Check sheet for the drawn part. Datum: minimum x, y, z corner. Units: mm. A direction names the side the tool comes from. Round coordinates to 2 decimals unless told otherwise and drop trailing zeros. Order: outer loops, then holes, each group sorted by start corner. A loop starts at its lowest first (then second) coordinate and runs counter-clockwise, first axis right, second up. Notation, with made-up numbers: (20, 30) -> (66, 30) arc R25 cw to (66, 60) -> close; hole circle Ø6 at (52, 80). An arc over 180 degrees is marked (long way). Answer as CSV lines item,"result". Start each with the question number.
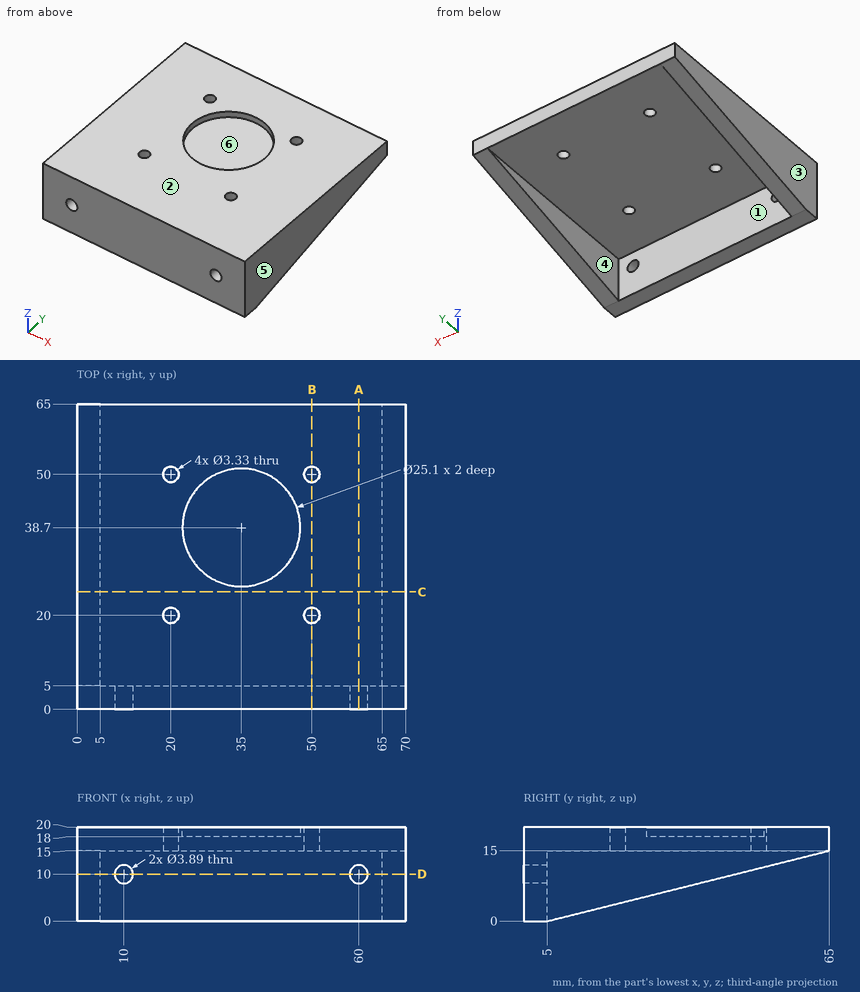
1) Section check B-B on x = 50. Record the cut outline in (y, z) (3 decimals), then the cut area to 3 significant figures.
2) Mould release check, pull along X, two halves, no side actions. Record for the marked faces 1, 2 and 3: released by +X, released by -X, zero draft, split by the parting line, or undercut.
3) Material ranges on line 1 along X through (y, z) = (20, 18.1) (3 decimals); line 2 along Y through (x, z) = (50, 18.9) (3 decimals); line 3 along Z through (x, y) = (60, 3.45) (3 decimals), recorded low to high.
4) Access from +Z, -Z, +X, -X, +Y, -Y to the whole of each face (thin tool, end or side, straight path). Record for the marked faces 4, 5 and 6.
5) Depth check by flat-ended pin: pin 1 Ø4 at (x, y) = (36.5, 30) entering from +Z; pin 2 Ø6 at (x, y) = (52, 56) entering from -Z; pin 3 Ø1 at (x, z) = (34, 4.5) entering from +Y; pin 4 Ø2.5 at (x, z) = (10, 10) entering from -Y. Enter the tip coordinate at first touch or a pass-through.
6) Section check D-D on z = 10. Record the cut outline in (x, y) (3 decimals), then the cut area to 3 significant figures.
7) Section check C-C on y = 25. Record the cut outline in (x, z), then the cut area to 3 significant figures.
8) Section check A-A on x = 60. Record the cut outline in (y, z) (3 decimals).
Solutions:
1,outline,"(0, 0) -> (5, 0) -> (5, 15) -> (18.335, 15) -> (18.335, 20) -> (0, 20) -> close; (21.665, 15) -> (48.335, 15) -> (48.335, 20) -> (21.665, 20) -> close; (51.665, 15) -> (65, 15) -> (65, 20) -> (51.665, 20) -> close"
1,area,"367 mm^2"
2,face 1,"undercut"
2,face 2,"zero draft"
2,face 3,"released by -X"
3,line 1,"x = 0 to 18.335, 21.665 to 48.335, 51.665 to 70"
3,line 2,"y = 0 to 18.335, 21.665 to 48.335, 51.665 to 65"
3,line 3,"z = 0 to 8.055, 11.945 to 20"
4,face 4,"-Z, +Y"
4,face 5,"+Z, -Z, +X, +Y, -Y"
4,face 6,"+Z"
5,pin 1,"stops at z = 18"
5,pin 2,"stops at z = 15"
5,pin 3,"stops at y = 5"
5,pin 4,"passes through"
6,outline,"(0, 0) -> (8.055, 0) -> (8.055, 5) -> (5, 5) -> (5, 45) -> (0, 45) -> close; (11.945, 0) -> (58.055, 0) -> (58.055, 5) -> (11.945, 5) -> close; (61.945, 0) -> (70, 0) -> (70, 45) -> (65, 45) -> (65, 5) -> (61.945, 5) -> close"
6,area,"711 mm^2"
7,outline,"(0, 5) -> (5, 5) -> (5, 15) -> (65, 15) -> (65, 5) -> (70, 5) -> (70, 20) -> (0, 20) -> close"
7,area,"450 mm^2"
8,outline,"(0, 0) -> (5, 0) -> (5, 8.055) -> (0, 8.055) -> close; (0, 11.945) -> (5, 11.945) -> (5, 15) -> (65, 15) -> (65, 20) -> (0, 20) -> close"
